from build123d import *

# Parameters (mm, degrees)
BOSS_EXTRUDE1_DEPTH  = 3
M6_CLEARANCE_HOLE1_D = 6.6
M6_CLEARANCE_HOLE2_D = 6.6


with BuildPart() as part:
    # Sketch1 → Boss-Extrude1 (new body)
    with BuildSketch(Plane.XY):
        with BuildLine():
            Line((26, 473), (49, 473))
            ThreePointArc((49, 473), (49.707106781, 473.292893219), (50, 474))
            Line((50, 474), (50, 497))
            ThreePointArc((50, 497), (50.292893219, 497.707106781), (51, 498))
            Line((51, 498), (94, 498))
            ThreePointArc((94, 498), (94.707106781, 497.707106781), (95, 497))
            Line((95, 497), (95, 473.5))
            ThreePointArc((95, 473.5), (95.292893219, 472.792893219), (96, 472.5))
            Line((96, 472.5), (109, 472.5))
            ThreePointArc((109, 472.5), (109.707106781, 472.207106781), (110, 471.5))
            Line((110, 471.5), (110, -23.5))
            ThreePointArc((110, -23.5), (109.707106781, -24.207106781), (109, -24.5))
            Line((109, -24.5), (96, -24.5))
            ThreePointArc((96, -24.5), (95.292893219, -24.792893219), (95, -25.5))
            Line((95, -25.5), (95, -49))
            ThreePointArc((95, -49), (94.707106781, -49.707106781), (94, -50))
            Line((94, -50), (51, -50))
            ThreePointArc((51, -50), (50.292893219, -49.707106781), (50, -49))
            Line((50, -49), (50, -26))
            ThreePointArc((50, -26), (49.707106781, -25.292893219), (49, -25))
            Line((49, -25), (26, -25))
            ThreePointArc((26, -25), (25.292893219, -24.707106781), (25, -24))
            Line((25, -24), (25, -1))
            ThreePointArc((25, -1), (24.707106781, -0.292893219), (24, 0))
            Line((24, 0), (1, 0))
            ThreePointArc((1, 0), (0.292893219, 0.292893219), (0, 1))
            Line((0, 1), (0, 447))
            ThreePointArc((0, 447), (0.292893219, 447.707106781), (1, 448))
            Line((1, 448), (24, 448))
            ThreePointArc((24, 448), (24.707106781, 448.292893219), (25, 449))
            Line((25, 449), (25, 472))
            ThreePointArc((25, 472), (25.292893219, 472.707106781), (26, 473))
        make_face()
    extrude(amount=BOSS_EXTRUDE1_DEPTH)

    # M6 Clearance Hole1 (through all)
    with Locations(Plane(origin=(0, 0, 0), x_dir=(-1, 0, 0), z_dir=(0, 0, -1))):
        with Locations((-72.5, -38.5), (-11.5, 12.5), (-11.5, 435.5), (-72.5, 486.5)):
            Hole(M6_CLEARANCE_HOLE1_D / 2)

    # M6 Clearance Hole2 (through all)
    with Locations(Plane(origin=(0, 0, 0), x_dir=(-1, 0, 0), z_dir=(0, 0, -1))):
        with Locations((-98.5, 224)):
            Hole(M6_CLEARANCE_HOLE2_D / 2)


solid = part.part
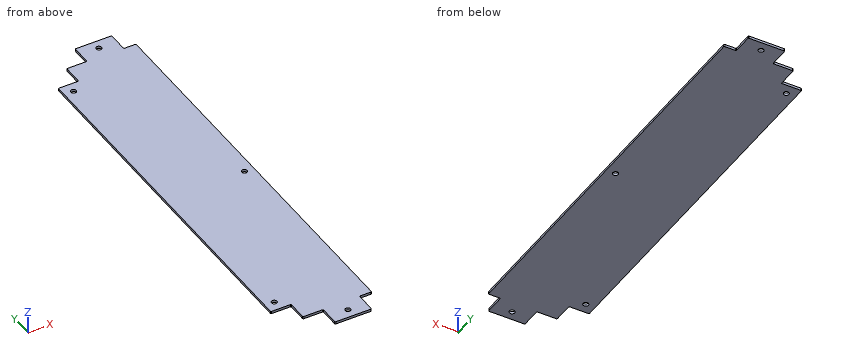
Geometry check sheet. Reference: the model listing, model coordinates, mm. Give positions to 0.01 mm unless a question says otherwise; leave off trailing zeros. Loops run counter-clockwise (first coordinate to the right, second up) from the corner with the lowest first, then second, coordinate; pieces in that order, holes last. Notation, with made-up numbers: (-40, 44) -> (-22, 44) arc R24 cw to (-22, 55) -> close; hole circle Ø10 at (65.25, -33.5). An arc over 180 degrees is marked (long way). Answer in a Markdown table with one row per item. Add a question column.
1) Gauge pin test, flat ends, axial feed: P1, Ø0.9, axis at x = 100.5, z = 2, coming from the -Y side; P2, Ø1.5, axis at x = 7.5, z = 1.5, coming from the -Y side; P3, Ø1.5, axis at y = 488, z = 1.5, coming from the -X side. Record the tip position at first contact, or that the pin passes through.
2) Material ranges on probe 1 along Y at (x, z) = (72.5, 0.8); probe 2 along Y at (x, z) = (11.5, 1.5); probe 3 along X at (y, z) = (486.5, 1.35), recorded low to high. Write a range as from..to.
3) Cross-section at B-B on x = 41. Record the boundary of the cut face in (y, z), and give its area (3 significant figures).
4) Cross-section at A-A on z = 2.35. State how many separate pieces and enclosed holes the cut face has, and give its area (3 significant figures).
Outcome:
| question | item | result |
|---|---|---|
| 1 | P1 | stops at y = -24.5 |
| 1 | P2 | stops at y = 0 |
| 1 | P3 | stops at x = 50 |
| 2 | probe 1 | y = -50..-41.8, -35.2..483.2, 489.8..498 |
| 2 | probe 2 | y = 0..9.2, 15.8..432.2, 438.8..448 |
| 2 | probe 3 | x = 50..69.2, 75.8..95 |
| 3 | outline | (-25, 0) -> (473, 0) -> (473, 3) -> (-25, 3) -> close |
| 3 | area | 1,490 mm^2 |
| 4 | separate pieces | 1 |
| 4 | enclosed holes | 5 |
| 4 | area | 55,600 mm^2 |
